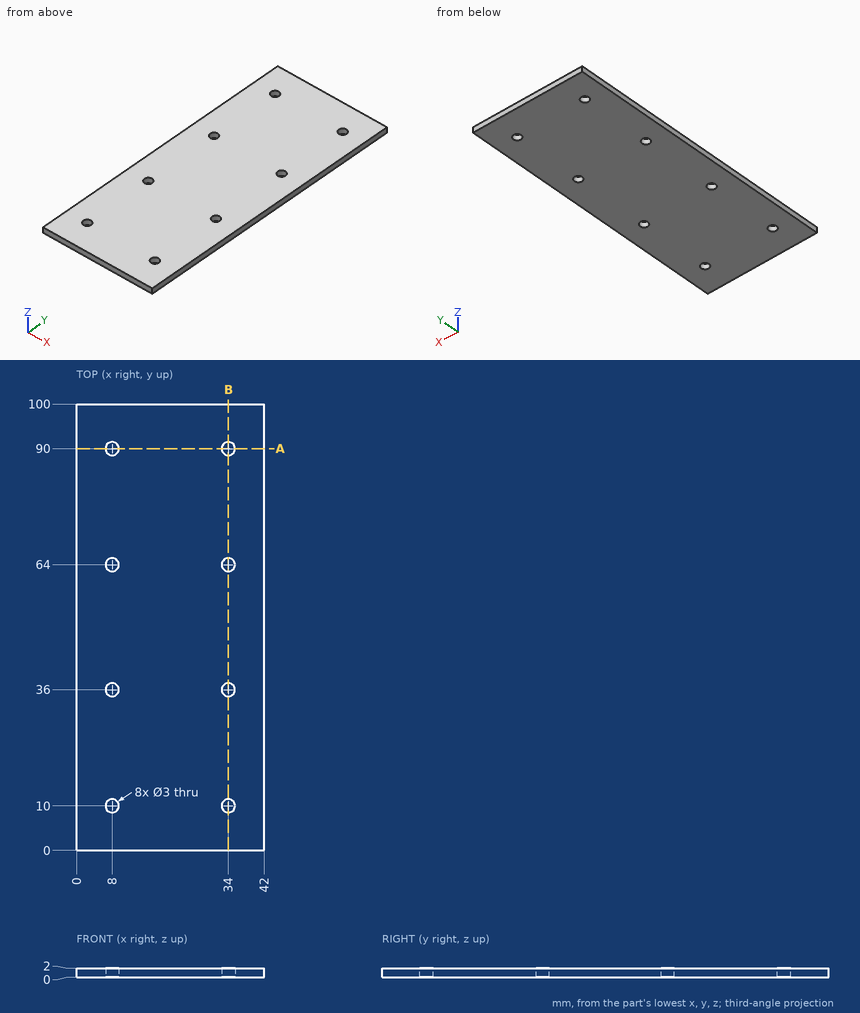
Answer from the drawing. Dimensions are ordinates in mm from the lowest x, y and z of the part. Coordinates: 2 decimals unless noted, no trailing zeros. Order: outer loops, then holes, each group sorted by start corner. A loop starts at its lowest first (then second) coordinate and runs counter-clockwise, first axis right, second up. Notation, with made-up numbers: (-23.5, 58) - (-8.5, 58) arc R23 ccw to (-8.5, 81) - close; hole circle Ø7 at (26, -33.5). An arc over 180 degrees is marked (long way). Use one line per item in the form item = value.
(1) Section A-A, the plane y = 90 is taken. Give the vertices of the cut face in (x, z).
Computed values:
outline = (0, 0) - (6.5, 0) - (6.5, 2) - (0, 2) - close; (9.5, 0) - (32.5, 0) - (32.5, 2) - (9.5, 2) - close; (35.5, 0) - (42, 0) - (42, 2) - (35.5, 2) - close
(2) Section B-B, the plane x = 34 is taken. Give the vertices of the cut face in (y, z), then the cut area to 3 significant figures.
Computed values:
outline = (0, 0) - (8.5, 0) - (8.5, 2) - (0, 2) - close; (11.5, 0) - (34.5, 0) - (34.5, 2) - (11.5, 2) - close; (37.5, 0) - (62.5, 0) - (62.5, 2) - (37.5, 2) - close; (65.5, 0) - (88.5, 0) - (88.5, 2) - (65.5, 2) - close; (91.5, 0) - (100, 0) - (100, 2) - (91.5, 2) - close
area = 176 mm²
(3) Straight lines are drawn through the part: L1, parallel to X at y = 64, z = 1; L2, parallel to Y at x = 8, z = 1.5; L3, parallel to X at y = 10.5, z = 0.35. For each, find the intervals that lie inside material, in ascending order.
Computed values:
L1 = 0 to 6.5, 9.5 to 32.5, 35.5 to 42
L2 = 0 to 8.5, 11.5 to 34.5, 37.5 to 62.5, 65.5 to 88.5, 91.5 to 100
L3 = 0 to 6.59, 9.41 to 32.59, 35.41 to 42
